Geometry: see drawing. Coordinates: mm, zero at the bounding-box minimum. Coordinates: 2 decimals unless noted, no trailing zeros. Use one line per item in the form item = value.
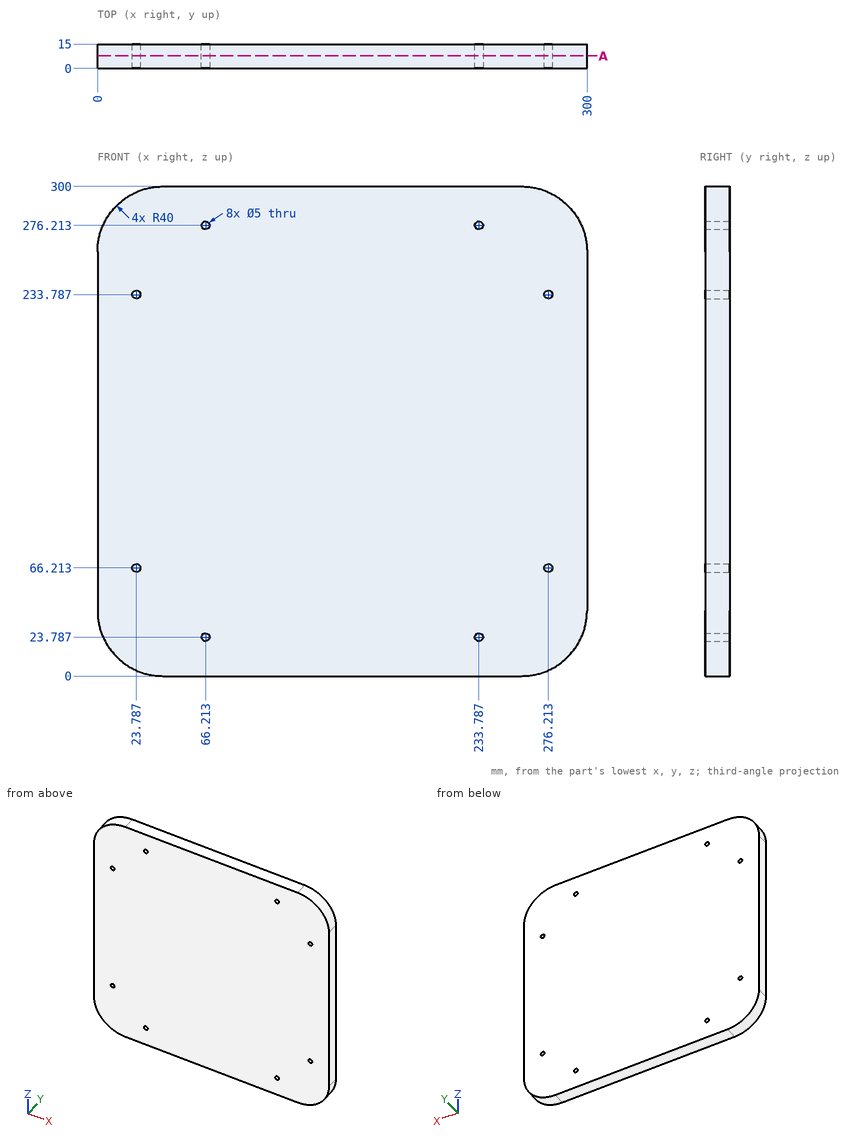
1) Section A-A, the plane y = 7.75. Give the number of separate pieces and of enclosed holes in the cut face, and give its area (3 significant figures).
Results found:
separate_pieces = 1
enclosed_holes = 8
area = 88,500 mm2
2) Contact query for a flat-ended pin moving along its axis: P1, Ø3, axis at x = 23.79, z = 233.79, coming from the -Y side. Output: stop coordinate, or through.
Results found:
P1 = through
3) Material intervals for probe 1 along Z at (x, y) = (67, 9.5); probe 2 along Z at (x, y) = (68, 9.5) (1 decimal); probe 3 along Z at (x, y) = (281, 11.75) (1 decimal), sorted ascending. Write a range as from..to.
Results found:
probe_1 = 0..21.41, 26.16..273.84, 278.59..300
probe_2 = 0..22, 25.5..274.5, 278..300
probe_3 = 6..294
